Build history of the part. All positions in model axes, mm. A direction names the side the tool comes from. Round coordinates to 2 decimals unless told otherwise and drop trailing zeros. Write each loop counter-clockwise with the first axis right and the second up, starting at its lowest first coordinate (ties: lowest second). Pieces come first, ordered by that corner, then holes.
1) Saw through at B-B (x = 15.5). Write the cut outline in (y, z) (3 decimals).
2) Flat gauge pins, fed straight in: pin 1 (4.5 mm diameter, centred on y = 5, z = 7.5, fed in from +X) (3 decimals); pin 2 (2.5 mm diameter, centred on x = -40, y = 1, fed in from +Z); pin 3 (1 mm diameter, centred on y = 3.5, z = 8.5, fed in from -X) (3 decimals). Where does each tip first touch, or does it go through?
3) Wall check: probe 1 along X at (y, z) = (-3.5, 5.25) (3 decimals); probe 2 along Y at (x, z) = (14, 8); probe 3 along Y at (x, z) = (-21.5, 8.25) (3 decimals). Give the ranges that are in metal, low to high.
4) Saw through at C-C (z = 3.75). Write the cut outline in (x, y) (3 decimals), plus the area to 3 significant figures.
5) Which spindle directions (+Z, -Z, +X, -X, +Y, -Y) get a long thin tool onto all of the face, cutting with end or side? Do faces 1 (the flat face through (-41, 0, 0.35)), 2 (the flat face through (41, 0, 0.35)), 3 (the flat face through (-1, 10.325, 4)). Say none if no direction does.
6) Saw through at A-A (y = 0). Write the cut outline in (x, z) (3 decimals), plus the area to 3 significant figures.
7) Saw through at D-D (y = -5.5). Write the cut outline in (x, z) (3 decimals), plus the area to 3 significant figures.
from build123d import *
from OCP.BRepFilletAPI import BRepFilletAPI_MakeChamfer

# Parameters (mm, degrees)
SKETCH1_W           = 77.11
SKETCH1_H           = 20.65
BOSS_EXTRUDE1_DEPTH = 14.97
CHAMFER1_SIZE       = 7
CHAMFER1_SIZE2      = 2
SKETCH2_W           = 5
SKETCH2_H           = 6.38
BOSS_EXTRUDE2_DEPTH = 0.35


with BuildPart() as part:
    # Sketch1 → Boss-Extrude1 (new body)
    with BuildSketch(Plane.XY):
        Rectangle(SKETCH1_W, SKETCH1_H)
    extrude(amount=BOSS_EXTRUDE1_DEPTH)

    # Chamfer1: one chamfer whose edges measure the first distance from different faces: ONE call of the kernel's chamfer builder (chamfer() names one face for all edges)
    chamfer1_edges_1 = [part.edges().sort_by_distance(p)[0] for p in [
        (0, -10.325, 14.97),
    ]]
    chamfer1_side_1 = [part.faces().sort_by_distance(p)[0] for p in [
        (0, -10.325, 7.485),
    ]]
    chamfer1_edges_2 = [part.edges().sort_by_distance(p)[0] for p in [
        (0, 10.325, 14.97),
    ]]
    chamfer1_side_2 = [part.faces().sort_by_distance(p)[0] for p in [
        (0, 10.325, 7.485),
    ]]
    chamfer1 = BRepFilletAPI_MakeChamfer(part.part.solid().wrapped)
    for e in chamfer1_edges_1:
        chamfer1.Add(CHAMFER1_SIZE, CHAMFER1_SIZE2, e.wrapped, chamfer1_side_1[0].wrapped)  # the first distance lies on this face
    for e in chamfer1_edges_2:
        chamfer1.Add(CHAMFER1_SIZE, CHAMFER1_SIZE2, e.wrapped, chamfer1_side_2[0].wrapped)  # the first distance lies on this face
    add(Compound.cast(chamfer1.Shape()), mode=Mode.REPLACE)

    # Sketch2 → Boss-Extrude2 (add)
    with BuildSketch(Plane(origin=(0, 0, 0), x_dir=(-1, 0, 0), z_dir=(0, 0, -1))):
        with Locations((-41.055, 0)):
            Rectangle(SKETCH2_W, SKETCH2_H)
        with Locations((41.055, 0)):
            Rectangle(SKETCH2_W, SKETCH2_H)
    extrude(amount=-BOSS_EXTRUDE2_DEPTH)


solid = part.part
Evaluation:
1. outline: (-10.325, 0) - (10.325, 0) - (10.325, 7.97) - (8.325, 14.97) - (-8.325, 14.97) - (-10.325, 7.97) - close
2. pin 1: stops at x = 38.555
2. pin 2: stops at z = 0.35
2. pin 3: stops at x = -38.555
3. probe 1: x = -38.555 to 38.555
3. probe 2: y = -10.32 to 10.32
3. probe 3: y = -10.245 to 10.245
4. outline: (-38.555, -10.325) - (38.555, -10.325) - (38.555, 10.325) - (-38.555, 10.325) - close
4. area: 1,590 mm2
5. face 1: +Z, -X, +Y, -Y
5. face 2: +Z, +X, +Y, -Y
5. face 3: +Z, -Z, +X, -X, +Y
6. outline: (-43.555, 0) - (43.555, 0) - (43.555, 0.35) - (38.555, 0.35) - (38.555, 14.97) - (-38.555, 14.97) - (-38.555, 0.35) - (-43.555, 0.35) - close
6. area: 1,160 mm2
7. outline: (-38.555, 0) - (38.555, 0) - (38.555, 14.97) - (-38.555, 14.97) - close
7. area: 1,150 mm2
